from build123d import *

# Parameters (mm, degrees)
BOSS_EXTRUDE1_DEPTH = 7
SKETCH2_R           = 2
BOSS_EXTRUDE2_DEPTH = 3


with BuildPart() as part:
    # Sketch1 → Boss-Extrude1 (new, symmetric)
    with BuildSketch(Plane(origin=(0, 0, 0), x_dir=(1, 0, 0), z_dir=(0, 1, 0))):
        Polygon((-1.154700538, 2), (-2.309401077, 0), (-1.154700538, -2), (1.154700538, -2), (2.309401077, 0), (1.154700538, 2), align=None)
    extrude(amount=BOSS_EXTRUDE1_DEPTH, both=True)

    # Sketch2 → Boss-Extrude2 (add)
    with BuildSketch(Plane(origin=(0, 7, 0), x_dir=(1, 0, 0), z_dir=(0, 1, 0))):
        with Locations(Location((0, 0, 0), (0, 0, 270))):
            Circle(SKETCH2_R)
    boss_extrude2 = extrude(amount=BOSS_EXTRUDE2_DEPTH)

    # Mirror1: Boss-Extrude2 across plane
    add(boss_extrude2.mirror(Plane.ZX))


solid = part.part
Design review of the part built by this model. Coordinates are the model's own, in mm. A direction names the side the tool comes from. Coordinates: 2 decimals unless noted, no trailing zeros. Loops run counter-clockwise (first coordinate to the right, second up) from the corner with the lowest first, then second, coordinate; pieces in that order, holes last. Notation, with made-up numbers: (-39.75, -15) - (-17.75, -15) arc R23 ccw to (-17.75, 2) - close; hole circle Ø3 at (33.25, 17). An arc over 180 degrees is marked (long way). Use CSV: the item, a comma, the result in double quotes. Start each with the question number.
1. Add section A-A on x = -0.7. Give the boundary of the cut face in (y, z).
2. To check wall thickness, follow probe 1 along X at (y, z) = (-1.5, 0.4); probe 2 along Z at (x, y) = (-2.05, 4.5); probe 3 along Z at (x, y) = (1.85, 6). State the ranges of each line that lie inside material, in increasing order.
3. For faces 1 (the cylindrical face through (-2, -8, 0)), 2 (the flat face through (0, -10, 0)), 3 (the cylindrical face through (-2, 8, 0)), list the 3-axis set-ups (+Z, -Z, +X, -X, +Y, -Y) from which the entire face can be reached by the end or side of a thin tool; tool diameter is ignored.
4. Clearance check with a flat-ended pin moving along its axis: pin 1 (0.6 mm diameter, centred on x = 2, z = 0.5, fed in from +Y). State where the tip first meets the part, or that it passes through.
5. Add section B-B on z = 1.5. Give the boundary of the cut face in (x, y).
6. Add section C-C on y = -4.75. Give the boundary of the cut face in (x, z).
Resolved:
1,outline,"(-10, -1.87) - (-7, -1.87) - (-7, -2) - (7, -2) - (7, -1.87) - (10, -1.87) - (10, 1.87) - (7, 1.87) - (7, 2) - (-7, 2) - (-7, 1.87) - (-10, 1.87) - close"
2,probe 1,"-2.08 to 2.08"
2,probe 2,"-0.45 to 0.45"
2,probe 3,"-0.8 to 0.8"
3,face 1,"-Y"
3,face 2,"+Z, -Z, +X, -X, -Y"
3,face 3,"+Y"
4,pin 1,"y = 10"
5,outline,"(-1.44, -7) - (-1.32, -7) - (-1.32, -10) - (1.32, -10) - (1.32, -7) - (1.44, -7) - (1.44, 7) - (1.32, 7) - (1.32, 10) - (-1.32, 10) - (-1.32, 7) - (-1.44, 7) - close"
6,outline,"(-2.31, 0) - (-1.15, -2) - (1.15, -2) - (2.31, 0) - (1.15, 2) - (-1.15, 2) - close"
